Here's how the part is built. I have some questions about the finished solid (model axes, mm). A direction names the side the tool comes from. Give positions to 0.01 mm unless a question says otherwise; leave off trailing zeros. Write each loop counter-clockwise with the first axis right and the second up, starting at its lowest first coordinate (ties: lowest second). Pieces come first, ordered by that corner, then holes. Notation, with made-up numbers: M -18,62 L 18,62 A22 cw 18,98 Z; hole C -4.75,74.5 d10. An arc over 180 degrees is marked long. Answer as CSV lines item,"result". Start each with the question number.
Q1. On a 3-axis mill with a long thin cutter (end or side, diameter ignored), from which of +Z, -Z, +X, -X, +Y, -Y can I reach the whole of each face in a straight line? I mean faces 1 (the flat face through (-3.25, 2, -5)), 2 (the flat face through (-3.25, 0.6, 4.1)), 3 (the flat face through (-1.517, 1, -8)), 4 (the flat face through (0, 2, 7.75)), 5 (the cylindrical face through (3.24, 2.27, 7.76)). Say none if no direction works.
Q2. Suppose I cut it at A-A (z = 6.5). Write out the boundary of the cut face in (x, y).
Q3. If I drill on line 1 along X through (y, z) = (0.4, 1.75); line 2 along Z through (x, y) = (0.25, 0.5); line 3 along Y through (x, z) = (-1.5, 4), over which ranges is the centre line in solid material (lowest first)?
Q4. Suppose I cut it at D-D (y = 3.1). Write out the boundary of the cut face in (x, z).
Q5. Thinking about a two-plate mould opening in X: for faces 6 (the flat face through (4.25, 1, 5)), 7 (the cylindrical face through (0.62, 0.51, 2.45)), 8 (the flat face through (3.8, 0.5, -0.25)), which applies, +X half, -X half, draft (parallel to the pull), parting line (faces both ways), or undercut?
Q6. Suppose I cut it at B-B (x = 0.25). Write out the boundary of the cut face in (y, z), then the cut area to 3 significant figures.
Q7. For pin 1 (1.8 mm diameter, centred on y = 2.5, z = 4, fed in from -X); pin 2 (0.8 mm diameter, centred on x = 4, y = 0.5, fed in from -Z); pin 3 (0.8 mm diameter, centred on y = 1, z = -8.5, fed in from +X), each with a flat end and sliding along its axis, tell me the tip position at first contact or that it passes through.
Q8. Suppose I cut it at C-C (z = 1.75). Write out the boundary of the cut face in (x, y), then the cut area to 3 significant figures.
```python
from build123d import *

# Parameters (mm, degrees)
SKETCH1_W                     = 8.5
SKETCH1_H                     = 17.5
BOSS_EXTRUDE1_DEPTH           = 3.5
SKETCH2_W                     = 6.5
SKETCH2_H                     = 15.5
CUT_EXTRUDE1_DEPTH            = 2.5
SKETCH3_R                     = 1.5
CUT_EXTRUDE2_DEPTH            = 2
SKETCH6_R                     = 0.5953125
CUT_EXTRUDE5_DEPTH            = 2.5
SKETCH7_R                     = 0.79375
CUT_EXTRUDE6_DEPTH            = 2
BOSS_EXTRUDE2_DEPTH           = 3.5
SKETCH14_W                    = 6.011083366
SKETCH14_H                    = 10.896717754
CUT_EXTRUDE8_DEPTH            = 0.75
TAP_DRILL_FOR_0_80_TAP1_D     = 1.19126
TAP_DRILL_FOR_0_80_TAP1_DEPTH = 7.11
TAP_DRILL_FOR_0_80_TAP1_TIP   = 0.357890611
CUT_EXTRUDE7_REACH            = 5.5
SKETCH15_W                    = 1
SKETCH15_H                    = 4
CUT_EXTRUDE9_DEPTH            = 2.5


with BuildPart() as part:
    # Sketch1 → Boss-Extrude1 (new body)
    with BuildSketch(Plane(origin=(0, 0, 0), x_dir=(1, 0, 0), z_dir=(0, 1, 0))):
        Rectangle(SKETCH1_W, SKETCH1_H)
    extrude(amount=BOSS_EXTRUDE1_DEPTH)

    # Sketch2 → Cut-Extrude1 (cut)
    with BuildSketch(Plane(origin=(0, 3.5, 0), x_dir=(1, 0, 0), z_dir=(0, 1, 0))):
        Rectangle(SKETCH2_W, SKETCH2_H)
    extrude(amount=-CUT_EXTRUDE1_DEPTH, mode=Mode.SUBTRACT)

    # Sketch3 → Cut-Extrude2 (cut, through all)
    with BuildSketch(Plane(origin=(0, 1, 0), x_dir=(1, 0, 0), z_dir=(0, 1, 0))):
        with Locations((0.25, -4.75)):
            Circle(SKETCH3_R)
    extrude(amount=-CUT_EXTRUDE2_DEPTH, mode=Mode.SUBTRACT)

    # Sketch6 → Cut-Extrude5 (cut)
    with BuildSketch(Plane(origin=(0, 3.5, 0), x_dir=(1, 0, 0), z_dir=(0, 1, 0))):
        with Locations((2.829050494, -7.329050494)):
            Circle(SKETCH6_R)
    extrude(amount=-CUT_EXTRUDE5_DEPTH, mode=Mode.SUBTRACT)

    # Sketch7 → Cut-Extrude6 (cut, through all)
    with BuildSketch(Plane(origin=(0, 1, 0), x_dir=(1, 0, 0), z_dir=(0, 1, 0))):
        with Locations((0.25, -1.75)):
            Circle(SKETCH7_R)
        with Locations((-1.625, -6.5)):
            Circle(SKETCH7_R)
        with Locations((2.125, -6.5)):
            Circle(SKETCH7_R)
    extrude(amount=-CUT_EXTRUDE6_DEPTH, mode=Mode.SUBTRACT)

    # Sketch9 → Boss-Extrude2 (add)
    with BuildSketch(Plane(origin=(0, 3.5, 0), x_dir=(1, 0, 0), z_dir=(0, 1, 0))):
        Polygon((-2.69064642, 9.789569053), (-4.770772156, 8.402818562), (-4.001541387, 7.248972409), (-3.411634369, 7.642243754), (-2.511322669, 8.242451554), (-1.921415651, 8.635722899), align=None)
    extrude(amount=-BOSS_EXTRUDE2_DEPTH)

    # Sketch14 → Cut-Extrude8 (cut)
    with BuildSketch(Plane(origin=(0, 3.5, 0), x_dir=(1, 0, 0), z_dir=(0, 1, 0))):
        with Locations((-3.25, 7.75)):
            Rectangle(SKETCH14_W, SKETCH14_H)
    extrude(amount=-CUT_EXTRUDE8_DEPTH, mode=Mode.SUBTRACT)

    # Tap Drill for #0-80 Tap1
    with Locations(Plane(origin=(-5.346153846, 0, -8.019230769), x_dir=(-0.832050294, 0, 0.554700196), z_dir=(-0.554700196, 0, -0.832050294))):
        with Locations((-1.941522729, 1.875)):
            Hole(TAP_DRILL_FOR_0_80_TAP1_D / 2, depth=TAP_DRILL_FOR_0_80_TAP1_DEPTH)
            with Locations((0, 0, -(TAP_DRILL_FOR_0_80_TAP1_DEPTH + TAP_DRILL_FOR_0_80_TAP1_TIP / 2))):  # 118° drill point
                Cone(0, TAP_DRILL_FOR_0_80_TAP1_D / 2, TAP_DRILL_FOR_0_80_TAP1_TIP, mode=Mode.SUBTRACT)

    # Sketch13 → Cut-Extrude7 (cut, up to next)
    with BuildSketch(Plane(origin=(0, 3.5, 0), x_dir=(1, 0, 0), z_dir=(0, 1, 0)), mode=Mode.PRIVATE) as cut_extrude7_sk1:
        Polygon((-3.249629447, -8.75), (-4.25, -8.75), (-4.25, 4.577582981), (-3.249629447, 3.077027151), align=None)
    cut_extrude7_tool1 = extrude(cut_extrude7_sk1.sketch, amount=-CUT_EXTRUDE7_REACH, mode=Mode.PRIVATE) & part.part
    add(cut_extrude7_tool1.solids().sort_by_distance((-3.759761, 3.5, 2.453888))[0], mode=Mode.SUBTRACT)
    # Sketch13 → Cut-Extrude7 (cut, up to next)
    with BuildSketch(Plane(origin=(0, 3.5, 0), x_dir=(1, 0, 0), z_dir=(0, 1, 0)), mode=Mode.PRIVATE) as cut_extrude7_sk2:
        Polygon((3.25, 0.25), (-1.517086772, 7.75), (-1.517086772, 8.75), (4.25, 8.75), (4.25, 0.25), align=None)
    cut_extrude7_tool2 = extrude(cut_extrude7_sk2.sketch, amount=-CUT_EXTRUDE7_REACH, mode=Mode.PRIVATE) & part.part
    add(cut_extrude7_tool2.solids().sort_by_distance((2.109513, 3.5, -5.504506))[0], mode=Mode.SUBTRACT)

    # Sketch15 → Cut-Extrude9 (cut)
    with BuildSketch(Plane(origin=(0, 3.5, 0), x_dir=(1, 0, 0), z_dir=(0, 1, 0))):
        with Locations((3.75, -1.75)):
            Rectangle(SKETCH15_W, SKETCH15_H)
    extrude(amount=-CUT_EXTRUDE9_DEPTH, mode=Mode.SUBTRACT)


solid = part.part
```
Resolved:
1,face 1,"+X, +Y"
1,face 2,"+Z, -X, +Y, -Y"
1,face 3,"-Z, +X, +Y, -Y"
1,face 4,"-X, +Y"
1,face 5,"+Y"
2,outline,"M -3.25,0 L -2.42,0 L -2.42,1 L -3.25,1 Z; M -0.83,0 L 1.33,0 L 1.33,1 L -0.83,1 Z; M 2.92,0 L 4.25,0 L 4.25,3.5 L 3.25,3.5 L 3.25,1 L 2.92,1 Z"
3,line 1,"-3.25 to -0.54, 1.04 to 4.25"
3,line 2,"-4.97 to 0.96, 2.54 to 3.25, 6.25 to 8.75"
3,line 3,"0 to 1"
4,outline,"M -3.25,7.75 L 2.41,7.75 A0.6 cw 3.25,6.91 L 3.25,3.75 L 4.25,3.75 L 4.25,8.75 L -3.25,8.75 Z"
5,face 6,"+X half"
5,face 7,"undercut"
5,face 8,"draft"
6,outline,"M 0,-4.97 L 1,-4.97 L 1,0.96 L 0,0.96 Z; M 0,2.54 L 1,2.54 L 1,3.25 L 0,3.25 Z; M 0,6.25 L 1,6.25 L 1,7.75 L 3.5,7.75 L 3.5,8.75 L 0,8.75 Z"
6,area,"11.6 mm^2"
7,pin 1,"x = 3.25"
7,pin 2,"z = -0.25"
7,pin 3,"x = -1.52"
8,outline,"M -3.25,0 L -0.54,0 L -0.54,1 L -3.25,1 Z; M 1.04,0 L 4.25,0 L 4.25,1 L 1.04,1 Z"
8,area,"5.91 mm^2"
